Autodesk Inventor part; units mm, degrees
ref_plane "YZ Plane" through (0, 0, 0) normal (1, 0, 0) x (0, 1, 0)
ref_plane "XZ Plane" through (0, 0, 0) normal (0, 1, 0) x (-1, 0, 0)
ref_plane "XY Plane" through (0, 0, 0) normal (0, 0, 1) x (1, 0, 0)
sketch "Sketch1" plane through (0, 0, 0) normal (0, 0, 1) x (1, 0, 0)
  line L0 (-6.5, 24) -> (6.5, 24)
  line L1 (6.5, 24) -> (6.5, -24)
  line L2 (6.5, -24) -> (-6.5, -24)
  line L3 (-6.5, -24) -> (-6.5, 24)
  line L4 (-6.5, 5) -> (-3.5, 5)
  line L5 (-3.5, 5) -> (-3.5, -5)
  line L6 (-3.5, -5) -> (-6.5, -5)
  line L7 (-6.5, -5) -> (-6.5, 5)
  line L8 (-3.5, 24) -> (3.5, 24)
  line L9 (3.5, 24) -> (3.5, 21)
  line L10 (3.5, 21) -> (-3.5, 21)
  line L11 (-3.5, 21) -> (-3.5, 24)
  line L12 (0, 0) -> (0.5, 0)
  line L13 (0, 0) -> (0, -2.6489)
  line L14 (6.5, 5) -> (3.5, 5)
  line L15 (3.5, 5) -> (3.5, -5)
  line L16 (3.5, -5) -> (6.5, -5)
  line L17 (3.5, -24) -> (3.5, -21)
  line L18 (3.5, -21) -> (-3.5, -21)
  line L19 (-3.5, -21) -> (-3.5, -24)
  line L20 (-3.5, -5) -> (-3.5, -24)
  line L21 (-3.5, 5) -> (-3.5, 24)
  line L22 (3.5, 24) -> (3.5, 5)
  line L23 (3.5, -5) -> (3.5, -24)
  point P0 (0, 24)
  point P1 (6.5, 0)
  point P2 (-3.5, 0)
  point P3 (0, 21)
  point P4 (0, -21)
  point P5 (6.5, 5)
  point P6 (6.5, -5)
  point P7 (3.5, 21)
  point P8 (3.5, -21)
  point P9 (3.5, 21)
  point P10 (-3.5, 21)
  point P11 (-3.5, -21)
  point P12 (3.5, -21)
  dimension "d0" = 48
  dimension "d1" = 13
  dimension "d2" = 3
  dimension "d3" = 10
  dimension "d4" = 7
  dimension "d5" = 3
extrude "Extrusion1" add sketch "Sketch1" along normal mid plane 3 contours L4 L5 L6 L3 | L10 L22 L15 L23 L18 L20 L5 L21 | L1 L16 L15 L14
properties part number "Side piece 2 2x"
Design review of the part built by this model. Coordinates are the model's own, in mm. A direction names the side the tool comes from. Round coordinates to 2 decimals unless told otherwise and drop trailing zeros. Loops run counter-clockwise (first coordinate to the right, second up) from the corner with the lowest first, then second, coordinate; pieces in that order, holes last. Notation, with made-up numbers: M 79.5,6.25 L 113.5,6.25 A19 ccw 113.5,30.25 Z; hole C -25.75,69 d1. An arc over 180 degrees is marked long. Answer as a JSON object with one key per item and string values.
Item 1: Wall thickness on L1, parallel to X at y = -17, z = 0.75; L2, parallel to Y at x = -4.5, z = 0: over which ranges is each line inside the solid? List them lowest first. Write a range as from..to.
Answer sheet:
{"L1": "x = -3.5..3.5", "L2": "y = -5..5"}
Item 2: Clearance check with flat-ended pins moving along their axes: P1, Ø1.5, axis at y = 13, z = 0, coming from the -X side; P2, Ø1.5, axis at y = 14.5, z = -0.5, coming from the +X side; P3, Ø0.9, axis at x = -5.5, z = 0.5, coming from the +Y side. State where each tip first meets the part, or that it passes through.
Answer sheet:
{"P1": "stops at x = -3.5", "P2": "stops at x = 3.5", "P3": "stops at y = 5"}
Item 3: We need section B-B on y = -10.5. Give the boundary of the cut face in (x, z).
Answer sheet:
{"outline": "M -3.5,-1.5 L 3.5,-1.5 L 3.5,1.5 L -3.5,1.5 Z"}
Item 4: Machinability: for faces 1 (the flat face through (5, 5, 0)), 2 (the flat face through (5, -5, 0)), 3 (the flat face through (-5, -5, 0)), which of the approach directions +Z, -Z, +X, -X, +Y, -Y give a long, thin tool a straight path to every point of the face, cutting with its end or side? Answer none if there is none.
Answer sheet:
{"face 1": "+Z, -Z, +X, +Y", "face 2": "+Z, -Z, +X, -Y", "face 3": "+Z, -Z, -X, -Y"}
Item 5: We need section A-A on z = -0.95. Give the boundary of the cut face in (x, y).
Answer sheet:
{"outline": "M -6.5,-5 L -3.5,-5 L -3.5,-21 L 3.5,-21 L 3.5,-5 L 6.5,-5 L 6.5,5 L 3.5,5 L 3.5,21 L -3.5,21 L -3.5,5 L -6.5,5 Z"}
Item 6: We need section C-C on x = 5. Give the boundary of the cut face in (y, z).
Answer sheet:
{"outline": "M -5,-1.5 L 5,-1.5 L 5,1.5 L -5,1.5 Z"}
